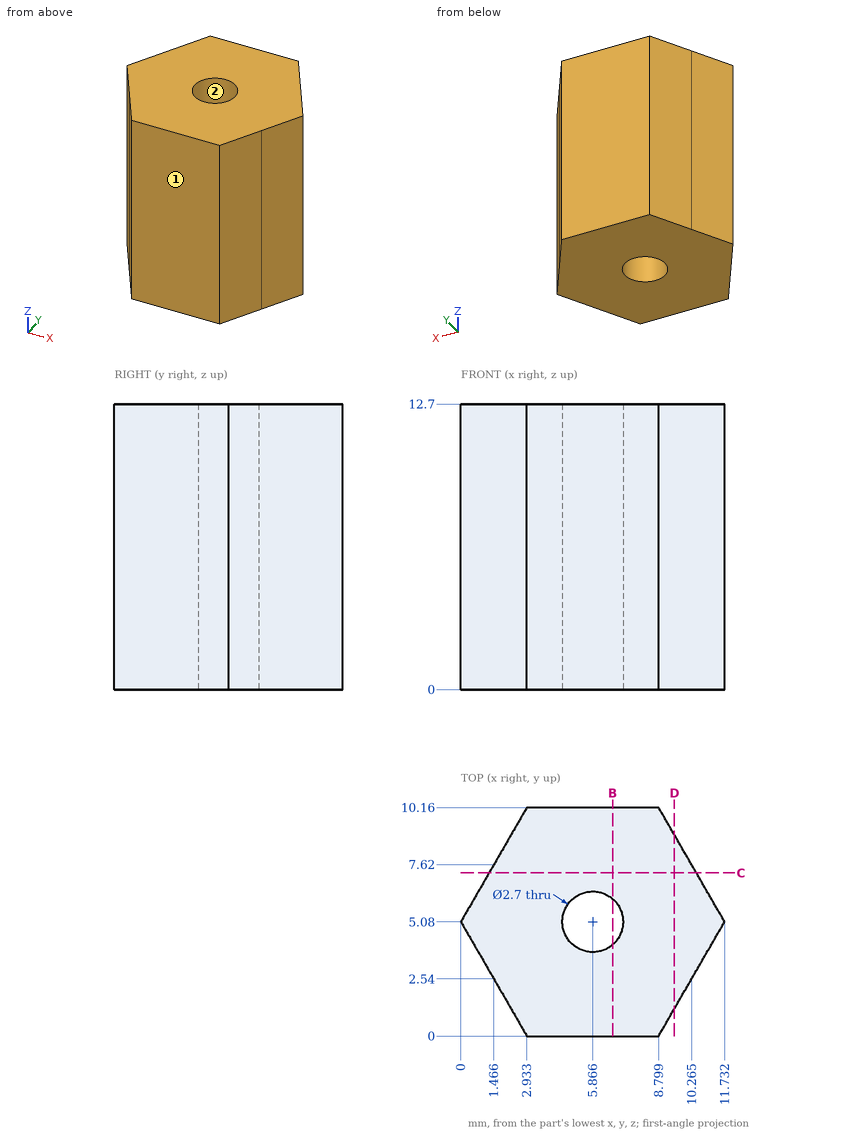
The figure shows three views and two pictorial views of one solid part (mm, origin at its lowest corner). Answer the questions. Give positions to 0.01 mm unless a question says otherwise; leave off trailing zeros. Write each loop counter-clockwise with the first axis right and the second up, starting at its lowest first coordinate (ties: lowest second). Pieces come first, ordered by that corner, then holes. Notation, with made-up numbers: (-25.5, 32.25) -> (24.5, 32.25) arc R21 ccw to (24.5, 47.25) -> close; hole circle Ø6 at (61, 13). An arc over 180 degrees is marked (long way). Answer as a JSON object with one key per item and string values.
1) For a pull along X with two mould halves and no side action, classify the marked faces 1 and 2 as pulls with the +X half, pulls with the -X half, needs draft (parallel to the pull), parting line crosses it, or undercut.
Findings below:
{"face 1": "needs draft", "face 2": "undercut"}
2) Section C-C on y = 7.25 is taken. Write down the section's boundary in (x, z), then the cut area to 3 significant figures.
Findings below:
{"outline": "(1.25, 0) -> (10.48, 0) -> (10.48, 12.7) -> (1.25, 12.7) -> close", "area": "117 mm^2"}
3) Section D-D on x = 9.5 is taken. Write down the section's boundary in (y, z) (1 decimal).
Findings below:
{"outline": "(1.2, 0) -> (8.9, 0) -> (8.9, 12.7) -> (1.2, 12.7) -> close"}
4) Flat-ended cylindrical pins translate along their axes: pin 1 Ø2.5 at (x, y) = (5.87, 5.08) entering from -Z; pin 2 Ø2 at (y, z) = (2, 6) entering from +X. Find the tip coordinate at first contact, or state that the pin passes through.
Findings below:
{"pin 1": "passes through", "pin 2": "stops at x = 10.53"}
5) Straight lines are drawn through the part: probe 1 along X at (y, z) = (6, 4.25) (1 decimal); probe 2 along X at (y, z) = (5.5, 3); probe 3 along Y at (x, z) = (6.25, 11.25) (1 decimal). For each, find the intervals that lie inside material, in ascending order. Write a range as from..to.
Findings below:
{"probe 1": "x = 0.5..4.9, 6.9..11.2", "probe 2": "x = 0.24..4.58, 7.15..11.49", "probe 3": "y = 0..3.8, 6.4..10.2"}
6) Section B-B on x = 6.75 is taken. Write down the section's boundary in (y, z), then the cut area to 3 significant figures.
Findings below:
{"outline": "(0, 0) -> (4.06, 0) -> (4.06, 12.7) -> (0, 12.7) -> close; (6.1, 0) -> (10.16, 0) -> (10.16, 12.7) -> (6.1, 12.7) -> close", "area": "103 mm^2"}
